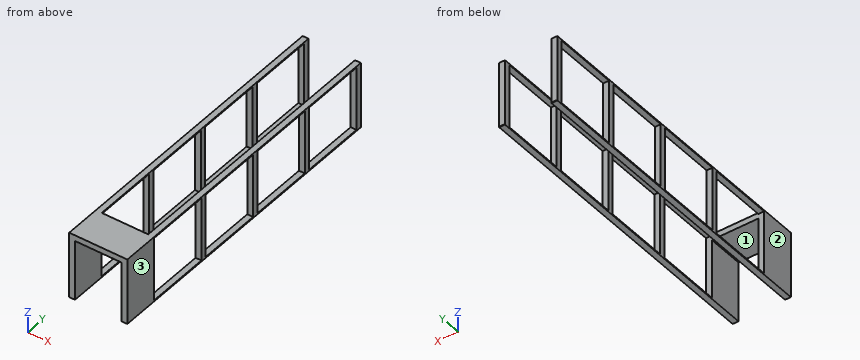
from build123d import *

# Parameters (mm, degrees)
SKETCH1_W            = 10
SKETCH1_H            = 2
BOSS_EXTRUDE1_DEPTH  = 112
SKETCH2_W            = 10
SKETCH2_H            = 2
BOSS_EXTRUDE2_DEPTH  = 480
SKETCH3_W            = 10
SKETCH3_H            = 2
BOSS_EXTRUDE3_DEPTH  = 90
SKETCH4_W            = 10
SKETCH4_H            = 2
BOSS_EXTRUDE4_DEPTH  = 102
SKETCH5_W            = 10
SKETCH5_H            = 2
BOSS_EXTRUDE5_DEPTH  = 480
SKETCH6_W            = 10
SKETCH6_H            = 10
BOSS_EXTRUDE6_DEPTH  = 110
SKETCH7_W            = 10
SKETCH7_H            = 10
BOSS_EXTRUDE7_DEPTH  = 110
SKETCH8_W            = 10
SKETCH8_H            = 10
BOSS_EXTRUDE8_DEPTH  = 110
SKETCH9_W            = 10
SKETCH9_H            = 10
BOSS_EXTRUDE9_DEPTH  = 110
BOSS_EXTRUDE10_DEPTH = 60
SKETCH12_W           = 10
SKETCH12_H           = 2
BOSS_EXTRUDE11_DEPTH = 542.116195333


with BuildPart() as part:
    # Sketch1 → Boss-Extrude1 (new body)
    with BuildSketch(Plane.XY):
        Rectangle(SKETCH1_W, SKETCH1_H)
    extrude(amount=BOSS_EXTRUDE1_DEPTH)

    # Sketch2 → Boss-Extrude2 (add)
    with BuildSketch(Plane(origin=(0, 1, 0), x_dir=(1, 0, 0), z_dir=(0, 1, 0))):
        with Locations((0, -111)):
            Rectangle(SKETCH2_W, SKETCH2_H)
    extrude(amount=BOSS_EXTRUDE2_DEPTH)

    # Sketch3 → Boss-Extrude3 (add)
    with BuildSketch(Plane(origin=(5, 0, 0), x_dir=(0, 0, -1), z_dir=(1, 0, 0))):
        with Locations((-107, 0)):
            Rectangle(SKETCH3_W, SKETCH3_H)
    extrude(amount=BOSS_EXTRUDE3_DEPTH)

    # Sketch4 → Boss-Extrude4 (add)
    with BuildSketch(Plane(origin=(0, 0, 102), x_dir=(-1, 0, 0), z_dir=(0, 0, -1))):
        with Locations((-90, 0)):
            Rectangle(SKETCH4_W, SKETCH4_H)
    extrude(amount=BOSS_EXTRUDE4_DEPTH)

    # Sketch5 → Boss-Extrude5 (add)
    with BuildSketch(Plane(origin=(0, 1, 0), x_dir=(1, 0, 0), z_dir=(0, 1, 0))):
        with Locations((90, -111)):
            Rectangle(SKETCH5_W, SKETCH5_H)
    extrude(amount=BOSS_EXTRUDE5_DEPTH)

    # Sketch6 → Boss-Extrude6 (add)
    with BuildSketch(Plane(origin=(0, 0, 110), x_dir=(-1, 0, 0), z_dir=(0, 0, -1))):
        with Locations((-90, 116)):
            Rectangle(SKETCH6_W, SKETCH6_H)
        with Locations((0, 116)):
            Rectangle(SKETCH6_W, SKETCH6_H)
    extrude(amount=BOSS_EXTRUDE6_DEPTH)

    # Sketch7 → Boss-Extrude7 (add)
    with BuildSketch(Plane(origin=(0, 0, 110), x_dir=(-1, 0, 0), z_dir=(0, 0, -1))):
        with Locations((-90, 236)):
            Rectangle(SKETCH7_W, SKETCH7_H)
        with Locations((0, 236)):
            Rectangle(SKETCH7_W, SKETCH7_H)
    extrude(amount=BOSS_EXTRUDE7_DEPTH)

    # Sketch8 → Boss-Extrude8 (add)
    with BuildSketch(Plane(origin=(0, 0, 110), x_dir=(-1, 0, 0), z_dir=(0, 0, -1))):
        with Locations((-90, 356)):
            Rectangle(SKETCH8_W, SKETCH8_H)
        with Locations((0, 356)):
            Rectangle(SKETCH8_W, SKETCH8_H)
    extrude(amount=BOSS_EXTRUDE8_DEPTH)

    # Sketch9 → Boss-Extrude9 (add)
    with BuildSketch(Plane(origin=(0, 0, 110), x_dir=(-1, 0, 0), z_dir=(0, 0, -1))):
        with Locations((-90, 476)):
            Rectangle(SKETCH9_W, SKETCH9_H)
        with Locations((0, 476)):
            Rectangle(SKETCH9_W, SKETCH9_H)
    extrude(amount=BOSS_EXTRUDE9_DEPTH)

    # Sketch11 → Boss-Extrude10 (add)
    with BuildSketch(Plane.XZ.offset(1)):
        Polygon((-5, 112), (-5, 0), (5, 0), (5, 102), (85, 102), (85, 0), (95, 0), (95, 112), align=None)
    extrude(amount=BOSS_EXTRUDE10_DEPTH)

    # Sketch12 → Boss-Extrude11 (add)
    with BuildSketch(Plane.XZ.offset(61)):
        with Locations((90, -1)):
            Rectangle(SKETCH12_W, SKETCH12_H)
        with Locations((0, -1)):
            Rectangle(SKETCH12_W, SKETCH12_H)
    extrude(amount=-BOSS_EXTRUDE11_DEPTH)


solid = part.part
Geometry: final body of the model. Coordinates: model frame, mm. Face numbers are marked on the shaded views. Give positions to 0.01 mm unless a question says otherwise; leave off trailing zeros. Loops run counter-clockwise (first coordinate to the right, second up) from the corner with the lowest first, then second, coordinate; pieces in that order, holes last. Notation, with made-up numbers: (8, 34) -> (47, 34) arc R16 cw to (47, 49) -> close; hole circle Ø7 at (69.25, 2.5). An arc over 180 degrees is marked (long way). Put each result on its own line as item: value.
1. Pull-direction query (X, two-part tool) for the marked faces 1, 2 and 3; classes: released by +X, released by -X, zero draft, split by the parting line, or undercut.
Taken from the geometry:
face 1: undercut
face 2: released by -X
face 3: released by +X
2. Cut plane C-C (x = 23.5). Return the cut outline in (y, z).
Taken from the geometry:
outline: (-61, 102) -> (1, 102) -> (1, 112) -> (-61, 112) -> close
3. Cut plane B-B (z = 81.5). Count the separate pieces of the cut face and the enclosed holes in it, plus the area to 3 significant figures.
Taken from the geometry:
separate pieces: 10
enclosed holes: 0
area: 2,040 mm2
4. Pin query (flat end, axial travel): P1, Ø8, axis at x = 1.5, z = 70.5, coming from the +Y side. Return the tip coordinate at first contact, or that it passes through.
Taken from the geometry:
P1: stops at y = 481
5. Ray query, line 1 along Y through (x, z) = (4.5, 8.5); line 2 along Z through (x, y) = (87, 264); line 3 along X through (y, z) = (-5, 63). Return the intervals inside material, ascending. Write a range as [from, to].
Taken from the geometry:
line 1: y = [-61, 1], [111, 121], [231, 241], [351, 361], [471, 481]
line 2: z = [-2, 0], [110, 112]
line 3: x = [-5, 5], [85, 95]
6. Cut plane A-A (y = 64). Return the cut outline in (x, z), plus the area to 3 significant figures.
Taken from the geometry:
outline: (-5, -2) -> (5, -2) -> (5, 0) -> (-5, 0) -> close; (-5, 110) -> (5, 110) -> (5, 112) -> (-5, 112) -> close; (85, -2) -> (95, -2) -> (95, 0) -> (85, 0) -> close; (85, 110) -> (95, 110) -> (95, 112) -> (85, 112) -> close
area: 80.0 mm2
